Could you check a few things on this model? Use its own coordinates, in mm. Face numbers are marked on the shaded views. Give positions to 0.01 mm unless a question says otherwise; leave off trailing zeros. Loops run counter-clockwise (first coordinate to the right, second up) from the corner with the lowest first, then second, coordinate; pieces in that order, holes last. Notation, with made-up numbers: M 24,74 L 57,74 A17 ccw 57,95 Z; hole C 10,-24 d4. An arc over 180 degrees is marked long. Use a Markdown table: item, result. Add a question column.
1) If I drill on line 1 along X through (y, z) = (1.5, 0.15); line 2 along Y through (x, z) = (13.5, -0.7); line 3 along Z through (x, y) = (-56, -5), over which ranges is the centre line in solid material (lowest first)? Write a range as [from, to].
2) Suppose I cut it at A-A on x = -42.5. List the corners of the cut face in (y, z) for me.
3) Will these pins go through, and if not, where does the flat tip stop? pin 1 Ø0.9 at (x, z) = (58, -1) entering from +Y; pin 2 Ø1 at (y, z) = (37.5, -1) entering from +X; pin 3 Ø0.5 at (y, z) = (-11, -1) entering from +X.
4) Suppose I cut it at B-B on y = 18. List the corners of the cut face in (x, z) for me, and give its area (3 significant figures).
5) We'd pull the mould along Y, two halves only. Please class the marked faces 1 and 2: +Y half, -Y half, draft (parallel to the pull), parting line (faces both ways), or undercut.
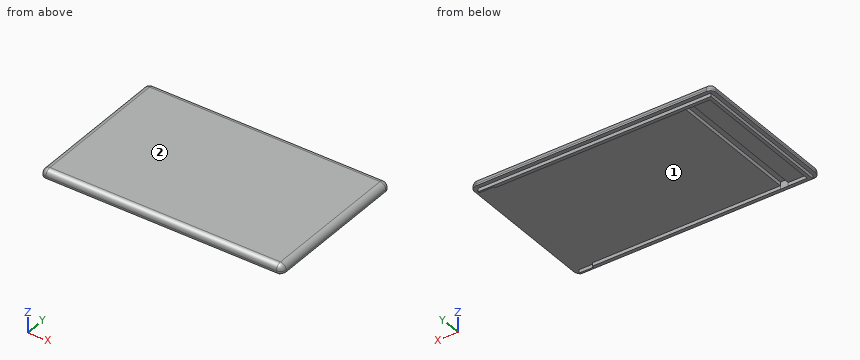
```python
from build123d import *

# Parameters (mm, degrees)
F0_W     = 128
F0_H     = 80
F1_DEPTH = 4
F2_W     = 7.8
F2_H     = 0.9
F2_W_2   = 1.8
F2_H_2   = 72.2
F3_DEPTH = 1.8
F4_W     = 4.2
F4_H     = 72.2
F5_DEPTH = 2
F6_W     = 4.2
F6_H     = 0.1
F7_DEPTH = 3.8
F8_R     = 3


with BuildPart() as f1:
    # F0 (on Top) → F1 (new body)
    with BuildSketch(Plane.XY):
        Rectangle(F0_W, F0_H)
    extrude(amount=F1_DEPTH)

    # F2 (on face) → F3 (join)
    with BuildSketch(Plane(origin=(0, 0, 0), x_dir=(1, 0, 0), z_dir=(0, 0, -1))):
        Polygon((53.5, 37.9), (-61.9, 37.9), (-61.9, 36.1), (-60.1, 36.1), (53.5, 36.1), (53.5, 37), align=None)
        with Locations((57.4, 37.45)):
            Rectangle(F2_W, F2_H)
        with Locations((-61, 0)):
            Rectangle(F2_W_2, F2_H_2)
        Polygon((-60.1, -36.1), (-61.9, -36.1), (-61.9, -37.9), (53.5, -37.9), (53.5, -37), (53.5, -36.1), align=None)
        with Locations((57.4, -37.45)):
            Rectangle(F2_W, F2_H)
    extrude(amount=F3_DEPTH)

    # F4 (on face) → F5 (cut)
    with BuildSketch(Plane(origin=(0, 0, 0), x_dir=(1, 0, 0), z_dir=(0, 0, -1))):
        with Locations((-48, 0)):
            Rectangle(F4_W, F4_H)
    extrude(amount=-F5_DEPTH, mode=Mode.SUBTRACT)

    # F6 (on face) → F7 (cut)
    with BuildSketch(Plane(origin=(0, 0, -1.8), x_dir=(1, 0, 0), z_dir=(0, 0, -1))):
        with Locations((-48, 36.15)):
            Rectangle(F6_W, F6_H)
        with Locations((-48, -36.15)):
            Rectangle(F6_W, F6_H)
    extrude(amount=-F7_DEPTH, mode=Mode.SUBTRACT)

    # F8
    f8_edges = [f1.edges().sort_by_distance(p)[0] for p in [
        (64, -40, 2),
        (64, 40, 2),
        (-64, 40, 2),
        (-64, -40, 2),
        (0, -40, 4),
        (-64, 0, 4),
        (0, 40, 4),
        (64, 0, 4),
    ]]
    fillet(f8_edges, radius=F8_R)


solid = f1.part
```
Answer block:
| question | item | result |
|---|---|---|
| 1 | line 1 | x = [-64, -50.1], [-45.9, 64] |
| 1 | line 2 | y = [-37.9, -36.1], [36.1, 37.9] |
| 1 | line 3 | z = [0, 4] |
| 2 | outline | M -40,0 L -37.9,0 L -37.9,-1.8 L -36.1,-1.8 L -36.1,0 L 36.1,0 L 36.1,-1.8 L 37.9,-1.8 L 37.9,0 L 40,0 L 40,1 A3 ccw 37,4 L -37,4 A3 ccw -40,1 Z |
| 3 | pin 1 | stops at y = 37.9 |
| 3 | pin 2 | stops at x = 61.3 |
| 3 | pin 3 | stops at x = -60.1 |
| 4 | outline | M -64,0 L -61.9,0 L -61.9,-1.8 L -60.1,-1.8 L -60.1,0 L -50.1,0 L -50.1,2 L -45.9,2 L -45.9,0 L 64,0 L 64,1 A3 ccw 61,4 L -61,4 A3 ccw -64,1 Z |
| 4 | area | 503 mm^2 |
| 5 | face 1 | undercut |
| 5 | face 2 | draft |
